Input: dimensioned drawing with shaded views. Units: mm. Origin: part minimum x, y, z. A direction names the side the tool comes from. Coordinates: 2 decimals unless noted, no trailing zeros. Order: outer loops, then holes, each group sorted by start corner. A loop starts at its lowest first (then second) coordinate and runs counter-clockwise, first axis right, second up. Notation, with made-up numbers: M -4,-9.5 L 38,-9.5 A24 cw 38,11.5 Z; hole C 2.25,32 d10. An arc over 180 degrees is marked long. Use CSV: the item, a comma, the result in double quotes. Start each with the question number.
1. Section query D-D on z = 7. Return the cut outline in (x, y).
2. Material intervals for line 1 (Y direction, x = 31.75, z = 11); line 2 (X direction, y = 31, z = 41) (1 decimal), sorted ascending.
3. Pull-direction query (Y, two-part tool) for the marked faces 3, 4 and 5; classes: pulls with the +Y half, pulls with the -Y half, needs draft (parallel to the pull), parting line crosses it, or undercut.
4. Set-up query: the marked faces 1 and 2. Return all of +Z, -Z, +X, -X, +Y, -Y with unobstructed straight access to the full face (end or side cutting, diameter ignored); none if empty.
5. Section query C-C on z = 37. Return the cut outline in (x, y).
6. Section query A-A on y = 31.75. Return the cut outline in (x, z).
7. First-contact query: P1, Ø2, axis at y = 13.5, z = 21.5, coming from the -X side (1 decimal); P2, Ø3, axis at y = 24.5, z = 35.5, coming from the -X side (3 decimals); P3, Ø4, axis at x = 19.5, y = 49.5, coming from the +Z side. Flat tips, straight axial feed; report the tip coordinate or a pass-through.
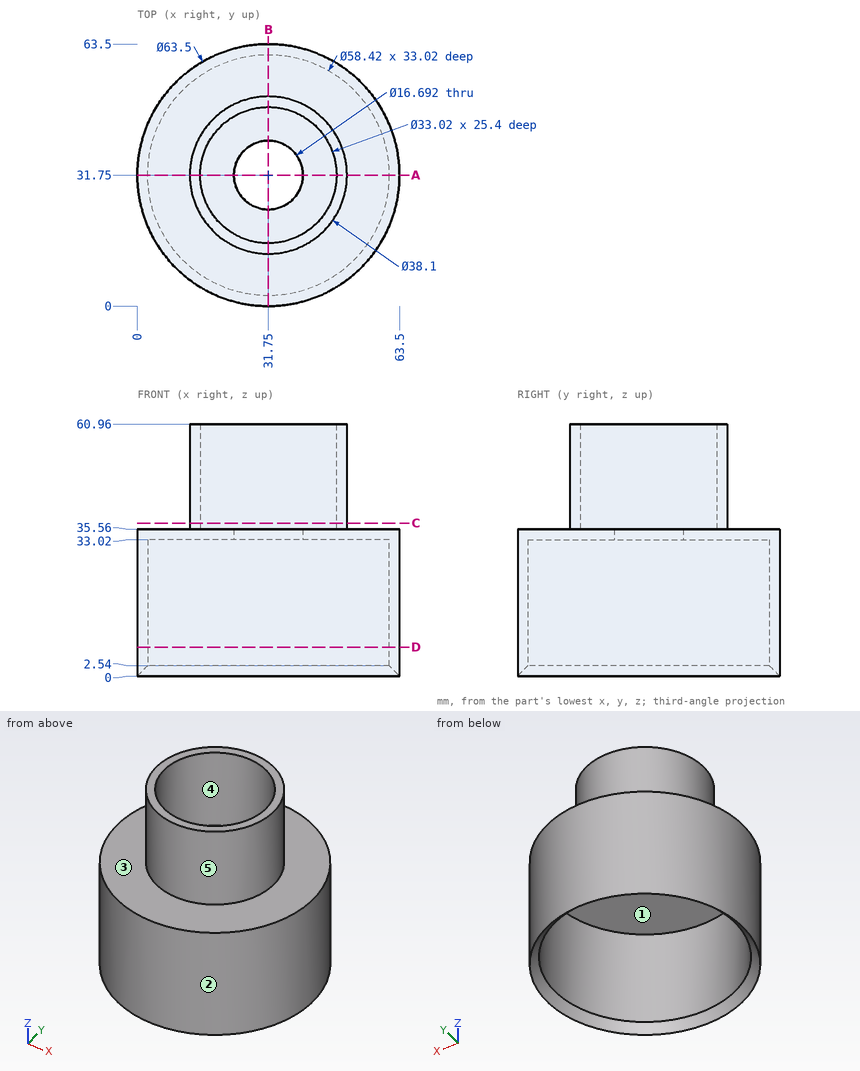
Results list:
1,outline,"C 31.75,31.75 d63.5; hole C 31.75,31.75 d58.42"
2,line 1,"y = 0 to 2.54, 60.96 to 63.5"
2,line 2,"x = 12.7 to 15.3, 48.2 to 50.8"
3,face 3,"needs draft"
3,face 4,"undercut"
3,face 5,"parting line crosses it"
4,face 1,"-Z"
4,face 2,"+Z, -Z"
5,outline,"C 31.75,31.75 d38.1; hole C 31.75,31.75 d33.02"
6,outline,"M 0,0 L 2.54,2.54 L 2.54,33.02 L 23.4,33.02 L 23.4,35.56 L 15.24,35.56 L 15.24,60.96 L 12.7,60.96 L 12.7,35.56 L 0,35.56 Z; M 40.1,33.02 L 60.96,33.02 L 60.96,2.54 L 63.5,0 L 63.5,35.56 L 50.8,35.56 L 50.8,60.96 L 48.26,60.96 L 48.26,35.56 L 40.1,35.56 Z"
7,P1,"stops at x = 5.1"
7,P2,"stops at x = 0.525"
7,P3,"stops at z = 35.56"
